from build123d import *

# Parameters (mm, degrees)
F0_R     = 6.0325
F0_R_2   = 2.8575
F6_DEPTH = 19.05


with BuildPart() as f2:
    # F2: sweep along a path in F1
    with BuildLine(Plane.XZ) as f2_path:
        Line((0, 0), (6.35, 0))
        ThreePointArc((6.35, 0), (10.8401280605, 1.8598719395), (12.7, 6.35))
        Line((12.7, 6.35), (12.7, 12.7))
    # F0 (on Right) → F2 (sweep)
    with BuildSketch(Plane.YZ):
        Circle(F0_R)
        Circle(F0_R_2, mode=Mode.SUBTRACT)
    sweep(path=f2_path.line)

    # F3 (on Front) → F4 (revolve)
    with BuildSketch(Plane.XZ):
        Polygon((10.0880871047, 18.624630657), (6.6675, 12.7), (9.8425, 12.7), (11.43, 15.449630657), (11.43, 18.624630657), align=None)
    revolve(axis=Axis((12.7, 0, 16.4198061287), (0, 0, 1)))

    # F5 (on Right) → F6 (join)
    with BuildSketch(Plane.YZ):
        with BuildLine():
            Line((0, -6.0325), (0, -2.8575))
            Line((0, -2.8575), (-3.175, -2.8575))
            Line((-3.175, -2.8575), (-3.175, -5.1293694788))
            ThreePointArc((-3.175, -5.1293694788), (-1.6504749118, -5.8023261556), (0, -6.0325))
        make_face()
        with BuildLine():
            Line((3.175, -2.8575), (0, -2.8575))
            Line((0, -2.8575), (0, -6.0325))
            ThreePointArc((0, -6.0325), (1.6504749118, -5.8023261556), (3.175, -5.1293694788))
            Line((3.175, -5.1293694788), (3.175, -2.8575))
        make_face()
        with BuildLine():
            ThreePointArc((3.175, -5.1293694788), (1.6504749118, -5.8023261556), (0, -6.0325))
            Line((0, -6.0325), (3.175, -6.0325))
            Line((3.175, -6.0325), (3.175, -5.1293694788))
        make_face()
        with BuildLine():
            Line((-3.175, -6.0325), (0, -6.0325))
            ThreePointArc((0, -6.0325), (-1.6504749118, -5.8023261556), (-3.175, -5.1293694788))
            Line((-3.175, -5.1293694788), (-3.175, -6.0325))
        make_face()
    extrude(amount=F6_DEPTH)


solid = f2.part
Build history of the part. All positions in model axes, mm. A direction names the side the tool comes from. Coordinates: 2 decimals unless noted, no trailing zeros. Write each loop counter-clockwise with the first axis right and the second up, starting at its lowest first coordinate (ties: lowest second). Pieces come first, ordered by that corner, then holes.
(1) Cut at C-C on z = 9. List the corners of the cut face in (x, y) (1 decimal).
(2) Mould opens along Z. For faces 1 (the flat face through (12, 3.175, -5)), 2 (the conical face through (11.29, 0.58, 15.01)), 3 (the cylindrical face through (9.867, -0.372, 9.569)), 4 (the conical face through (15.9, -0.1, 17.6)) say: pulls with the +Z half, pulls with the -Z half, needs draft (parallel to the pull), parting line crosses it, or undercut.
(3) Pin check, flat tips, straight feed: pin 1 Ø4.5 at (y, z) = (0, 0) entering from +X; pin 2 Ø4 at (x, z) = (5.5, 9.5) entering from +Y; pin 3 Ø3.5 at (x, z) = (13, -4) entering from +Y; pin 4 Ø1.5 at (y, z) = (0, 3) entering from -X. Stop position of each tip, or through.
(4) 3-axis set-ups, long thin cutter, end or side, ignore diameter. For faces 5 (the flat face through (0, 3, -1)), 6 (the cylindrical face through (13.97, -0.06, 17.06)), 7 (the flat face through (14, -1, 18.625)), 8 (the cylindrical face through (3.219, 2.726, 0.858)), 9 (the flat face through (12, -3.175, -5)): which of +Z, -Z, +X, -X, +Y, -Y reach the whole face in a straight line?
(5) Drill centre lines: line 1 (X direction, y = 0, z = 10.75); line 2 (Y direction, x = 12.7, z = 10.5); line 3 (X direction, y = -1.25, z = 9.25). Where is each one in solid material? Low to high.
(6) Cut at B-B on x = 3.75. List the corners of the cut face in (y, z) (1 decimal), and give its area (3 significant figures).
Working result:
1. outline: circle Ø12.1 at (12.7, 0); hole circle Ø5.7 at (12.7, 0)
2. face 1: needs draft
2. face 2: undercut
2. face 3: undercut
2. face 4: pulls with the +Z half
3. pin 1: stops at x = 18.03
3. pin 2: stops at y = 3.06
3. pin 3: stops at y = 4.33
3. pin 4: stops at x = 0
4. face 5: +Z, -Z, -X, +Y, -Y
4. face 6: +Z
4. face 7: +Z, +X, -X, +Y, -Y
4. face 8: -X
4. face 9: -Z, +X, -Y
5. line 1: x = 6.67 to 9.84, 15.56 to 18.73
5. line 2: y = -6.03 to -2.86, 2.86 to 6.03
5. line 3: x = 6.8 to 10.13, 15.27 to 18.6
6. outline: (-3.2, -6) - (3.2, -6) - (3.2, -5.1) arc R6 ccw (long way) to (-3.2, -5.1) - close; hole circle Ø5.7 at (0, 0)
6. area: 90.5 mm2
